```python
from build123d import *

# Parameters (mm, degrees)
SKETCH1_W           = 129.7
SKETCH1_H           = 180
SKETCH1_R           = 2.5
SKETCH1_R_2         = 3.6
BOSS_EXTRUDE1_DEPTH = 5
FILLET1_R           = 3


with BuildPart() as part:
    # Sketch1 → Boss-Extrude1 (new body)
    with BuildSketch(Plane.XY):
        with Locations((64.85, 90)):
            Rectangle(SKETCH1_W, SKETCH1_H)
        with Locations((15, 15)):
            Circle(SKETCH1_R, mode=Mode.SUBTRACT)
        with Locations((15, 165)):
            Circle(SKETCH1_R, mode=Mode.SUBTRACT)
        with Locations((114.7, 165)):
            Circle(SKETCH1_R_2, mode=Mode.SUBTRACT)
        with Locations((114.7, 15)):
            Circle(SKETCH1_R_2, mode=Mode.SUBTRACT)
        with Locations((34.85, 140)):
            Circle(SKETCH1_R, mode=Mode.SUBTRACT)
        with Locations((64.85, 140)):
            Circle(SKETCH1_R, mode=Mode.SUBTRACT)
        with Locations((94.85, 140)):
            Circle(SKETCH1_R, mode=Mode.SUBTRACT)
        with Locations((34.85, 40)):
            Circle(SKETCH1_R, mode=Mode.SUBTRACT)
        with Locations((64.85, 40)):
            Circle(SKETCH1_R, mode=Mode.SUBTRACT)
        with Locations((94.85, 40)):
            Circle(SKETCH1_R, mode=Mode.SUBTRACT)
        with Locations((94.85, 120)):
            Circle(SKETCH1_R, mode=Mode.SUBTRACT)
        with Locations((64.85, 120)):
            Circle(SKETCH1_R, mode=Mode.SUBTRACT)
        with Locations((34.85, 120)):
            Circle(SKETCH1_R, mode=Mode.SUBTRACT)
        with Locations((34.85, 60)):
            Circle(SKETCH1_R, mode=Mode.SUBTRACT)
        with Locations((64.85, 60)):
            Circle(SKETCH1_R, mode=Mode.SUBTRACT)
        with Locations((94.85, 60)):
            Circle(SKETCH1_R, mode=Mode.SUBTRACT)
    extrude(amount=BOSS_EXTRUDE1_DEPTH)

    # Fillet1
    fillet1_edges = [part.edges().sort_by_distance(p)[0] for p in [
        (0, 180, 2.5),
        (129.7, 180, 2.5),
        (129.7, 0, 2.5),
        (0, 0, 2.5),
    ]]
    fillet(fillet1_edges, radius=FILLET1_R)


solid = part.part
```
Could you check a few things on this model? Use its own coordinates, in mm. Coordinates: 2 decimals unless noted, no trailing zeros. Write each loop counter-clockwise with the first axis right and the second up, starting at its lowest first coordinate (ties: lowest second). Pieces come first, ordered by that corner, then holes. Notation, with made-up numbers: (8.25, 52.25) -> (17.25, 52.25) arc R20 cw to (17.25, 89.25) -> close; hole circle Ø6 at (8.5, -36.75). An arc over 180 degrees is marked (long way). Write item = value, one per line. Start each with the question number.
(1) I need wall thicknesses on line 1 (Y direction, x = 94.5, z = 3.95); line 2 (X direction, y = 140, z = 3.25); line 3 (Y direction, x = 114.7, z = 2.7). Which ranges of each line are inside material? Lowest first, please. Write a range as [from, to].
(2) I want a section at D-D (y = 15). Please give me the cut outline in (x, z).
(3) I want a section at B-B (z = 3.5). Give the number of separate pieces and of enclosed holes in the cut face, plus the area to 3 significant figures.
(4) We'd pull the mould along X, two halves only. Please class faces 1 (the face through (64, 91, 0)), 2 (the face through (129.7, 89, 2)), 3 (the face through (118.025, 13.621, 2.465)), 4 (the face through (96.19, 142.11, 2.46)): released by +X, released by -X, zero draft, split by the parting line, or undercut.
(5) Will this pin go through, and if not, where does the flat tip stop? pin 1 (8 mm diameter, centred on x = 94.85, y = 140, fed in from +Z).
(6) I want a section at C-C (x = 114.7). Please give me the cut outline in (y, z).
(7) I want a section at A-A (y = 120). Please give me the cut outline in (x, z).
Result set:
q1.line_1 = [0, 37.52], [42.48, 57.52], [62.48, 117.52], [122.48, 137.52], [142.48, 180]
q1.line_2 = [0, 32.35], [37.35, 62.35], [67.35, 92.35], [97.35, 129.7]
q1.line_3 = [0, 11.4], [18.6, 161.4], [168.6, 180]
q2.outline = (0, 0) -> (12.5, 0) -> (12.5, 5) -> (0, 5) -> close; (17.5, 0) -> (111.1, 0) -> (111.1, 5) -> (17.5, 5) -> close; (118.3, 0) -> (129.7, 0) -> (129.7, 5) -> (118.3, 5) -> close
q3.separate_pieces = 1
q3.enclosed_holes = 16
q3.area = 23,000 mm2
q4.face_1 = zero draft
q4.face_2 = released by +X
q4.face_3 = undercut
q4.face_4 = undercut
q5.pin_1 = 5
q6.outline = (0, 0) -> (11.4, 0) -> (11.4, 5) -> (0, 5) -> close; (18.6, 0) -> (161.4, 0) -> (161.4, 5) -> (18.6, 5) -> close; (168.6, 0) -> (180, 0) -> (180, 5) -> (168.6, 5) -> close
q7.outline = (0, 0) -> (32.35, 0) -> (32.35, 5) -> (0, 5) -> close; (37.35, 0) -> (62.35, 0) -> (62.35, 5) -> (37.35, 5) -> close; (67.35, 0) -> (92.35, 0) -> (92.35, 5) -> (67.35, 5) -> close; (97.35, 0) -> (129.7, 0) -> (129.7, 5) -> (97.35, 5) -> close
